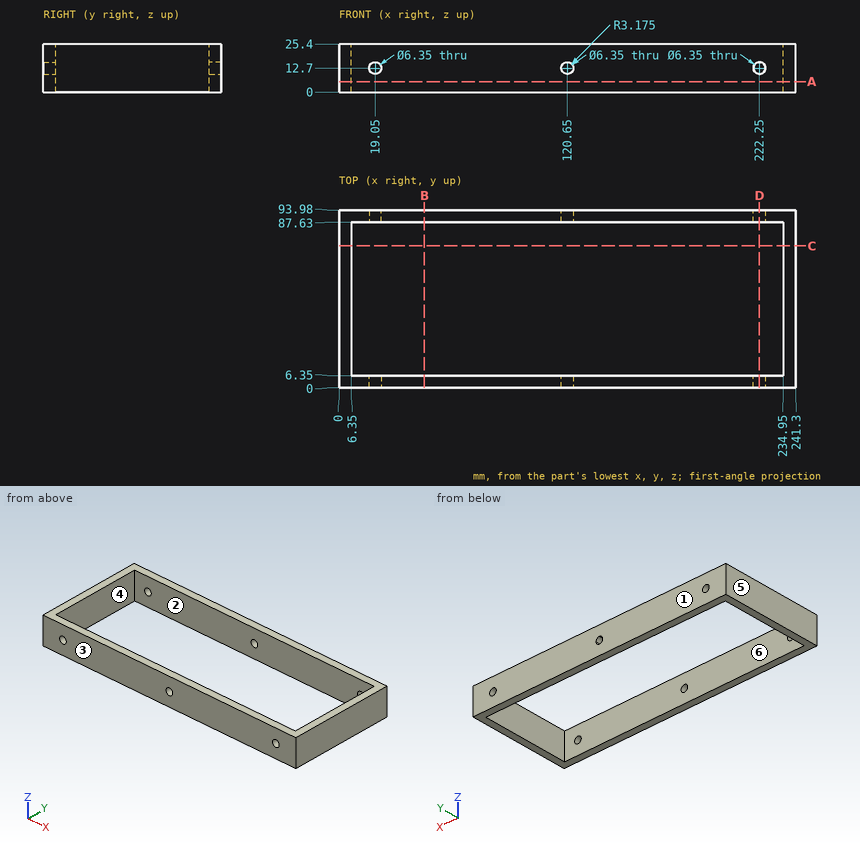
The figure shows three views and two pictorial views of one solid part (mm, origin at its lowest corner). Answer the questions. A direction names the side the tool comes from. Round coordinates to 2 decimals unless told otherwise and drop trailing zeros. Order: outer loops, then holes, each group sorted by start corner. A loop starts at its lowest first (then second) coordinate and runs counter-clockwise, first axis right, second up. Notation, with made-up numbers: (43.25, 30.5) - (52.25, 30.5) arc R20 cw to (52.25, 64.5) - close; hole circle Ø6 at (-6, -18). An arc over 180 degrees is marked (long way). Write item = value, one per line. Start each with the question number.
1) For the marked faces 5 and 6, determine the directions among +Z, -Z, +X, -X, +Y, -Y from which every point of the face is accessible in a straight line to the end or side of a thin tool.
2) Section C-C, the plane y = 75 is taken. Write down the section's boundary in (x, z), plus the area to 3 significant figures.
3) Section B-B, the plane x = 45 is taken. Write down the section's boundary in (y, z), plus the area to 3 significant figures.
4) For a pull along Y with two mould halves and no side action, classify the marked faces 1, 2, 3 and 4 as released by +Y, released by -Y, zero draft, split by the parting line, or undercut.
5) Section D-D, the plane x = 222.25 is taken. Write down the section's boundary in (y, z) (3 decimals).
6) Section A-A, the plane z = 5.5 is taken. Write down the section's boundary in (x, y), plus the area to 3 significant figures.
7) Straight lines are drawn through the part: L1, parallel to X at y = 5, z = 12.7 (3 decimals); L2, parallel to Y at x = 14.5, z = 20.25; L3, parallel to X at y = 22, z = 20.5. For each, find the intervals that lie inside material, in ascending order.
Results list:
q1.face_5 = +Z, -Z, -X, +Y, -Y
q1.face_6 = +Z, -Z
q2.outline = (0, 0) - (6.35, 0) - (6.35, 25.4) - (0, 25.4) - close; (234.95, 0) - (241.3, 0) - (241.3, 25.4) - (234.95, 25.4) - close
q2.area = 323 mm^2
q3.outline = (0, 0) - (6.35, 0) - (6.35, 25.4) - (0, 25.4) - close; (87.63, 0) - (93.98, 0) - (93.98, 25.4) - (87.63, 25.4) - close
q3.area = 323 mm^2
q4.face_1 = released by +Y
q4.face_2 = undercut
q4.face_3 = released by -Y
q4.face_4 = undercut
q5.outline = (0, 0) - (6.35, 0) - (6.35, 9.525) - (0, 9.525) - close; (0, 15.875) - (6.35, 15.875) - (6.35, 25.4) - (0, 25.4) - close; (87.63, 0) - (93.98, 0) - (93.98, 9.525) - (87.63, 9.525) - close; (87.63, 15.875) - (93.98, 15.875) - (93.98, 25.4) - (87.63, 25.4) - close
q6.outline = (0, 0) - (241.3, 0) - (241.3, 93.98) - (0, 93.98) - close; hole (6.35, 6.35) - (234.95, 6.35) - (234.95, 87.63) - (6.35, 87.63) - close
q6.area = 4,100 mm^2
q7.L1 = 0 to 15.875, 22.225 to 117.475, 123.825 to 219.075, 225.425 to 241.3
q7.L2 = 0 to 6.35, 87.63 to 93.98
q7.L3 = 0 to 6.35, 234.95 to 241.3
